Read the model definition and answer for the solid it produces. Units are mm, in the model's axes. Face numbers are marked on the shaded views. A direction names the side the tool comes from. Give positions to 0.01 mm unless a question says otherwise; leave off trailing zeros. Write each loop counter-clockwise with the first axis right and the second up, starting at its lowest first coordinate (ties: lowest second). Pieces come first, ordered by that corner, then holes.
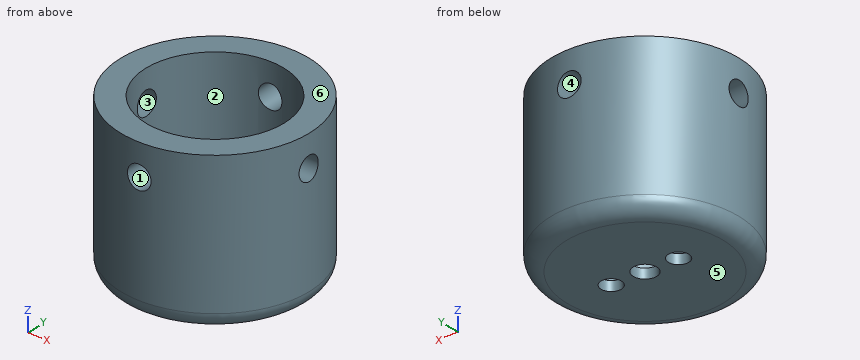
```python
from build123d import *

# Parameters (mm, degrees)
F0_R          = 30.48
F1_DEPTH      = 50.8
F2_R          = 3.81
F3_DEPTH      = 50.801
F4_R          = 3.81
F5_DEPTH      = 30.481
F5_DEPTH_BACK = 30.481
F6_R          = 3.81
F7_DEPTH      = 30.4810001
F7_DEPTH_BACK = 30.4810001
F8_R          = 3.302
F9_DEPTH      = 50.8010001
F10_R         = 22.352
F11_DEPTH     = 47.625
F12_R         = 5.08


with BuildPart() as f1:
    # F0 (on Top) → F1 (new body)
    with BuildSketch(Plane.XY):
        Circle(F0_R)
    extrude(amount=-F1_DEPTH)

    # F2 (on face) → F3 (cut, through all)
    with BuildSketch(Plane(origin=(0, 0, -50.8), x_dir=(1, 0, 0), z_dir=(0, 0, -1))):
        Circle(F2_R)
    extrude(amount=-F3_DEPTH, mode=Mode.SUBTRACT)

    # F4 (on Right) → F5 (cut, two sides)
    with BuildSketch(Plane.YZ) as f5_sk:
        with Locations((0, -10.16)):
            Circle(F4_R)
    extrude(amount=-F5_DEPTH, mode=Mode.SUBTRACT)
    extrude(f5_sk.sketch, amount=F5_DEPTH_BACK, mode=Mode.SUBTRACT)

    # F6 (on Front) → F7 (cut, two sides)
    with BuildSketch(Plane.XZ) as f7_sk:
        with Locations((0, -10.16)):
            Circle(F6_R)
    extrude(amount=-F7_DEPTH, mode=Mode.SUBTRACT)
    extrude(f7_sk.sketch, amount=F7_DEPTH_BACK, mode=Mode.SUBTRACT)

    # F8 (on face) → F9 (cut, through all)
    with BuildSketch(Plane(origin=(0, 0, -50.8), x_dir=(1, 0, 0), z_dir=(0, 0, -1))):
        with Locations((10.922, 0)):
            Circle(F8_R)
        with Locations((-10.8710342307, 0)):
            Circle(F8_R)
    extrude(amount=-F9_DEPTH, mode=Mode.SUBTRACT)

    # F10 (on face) → F11 (cut)
    with BuildSketch(Plane.XY):
        Circle(F10_R)
    extrude(amount=-F11_DEPTH, mode=Mode.SUBTRACT)

    # F12
    f12_edges = [f1.edges().sort_by_distance(p)[0] for p in [
        (-30.48, 0, -50.8),
    ]]
    fillet(f12_edges, radius=F12_R)


solid = f1.part
```
Item 1: Which of the six approach directions +Z, -Z, +X, -X, +Y, -Y give full straight-line access (tool end or side, diameter ignored) to the marked faces 1 and 2?
Result set:
face 1: +Y, -Y
face 2: +Z
Item 2: Section D-D (z = -17.5) is taken. Write down the section's boundary in (x, y).
Result set:
outline: circle Ø60.96 at (0, 0); hole circle Ø44.7 at (0, 0)
Item 3: Each of these flat-tipped pins is pushed along its axis until it touches: pin 1 Ø1.5 at (x, z) = (7, -26.5) entering from -Y; pin 2 Ø9 at (x, z) = (0, -10.16) entering from -Y; pin 3 Ø3 at (x, z) = (-5, -11.5) entering from -Y; pin 4 Ø7.5 at (x, y) = (10.922, 0) entering from +Z (3 decimals). Where does it stop, or does it pass through?
Result set:
pin 1: stops at y = -29.83
pin 2: stops at y = -30.48
pin 3: stops at y = -30.28
pin 4: stops at z = -47.625
Item 4: Section C-C (z = -10.16) is taken. Write down the section's boundary in (x, y), and give its area (3 significant figures).
Result set:
outline: (-30.24, -3.81) arc R30.48 ccw to (-3.81, -30.24) - (-3.81, -22.02) arc R22.35 cw to (-22.02, -3.81) - close; (-30.24, 3.81) - (-22.02, 3.81) arc R22.35 cw to (-3.81, 22.02) - (-3.81, 30.24) arc R30.48 ccw to start; (3.81, -30.24) arc R30.48 ccw to (30.24, -3.81) - (22.02, -3.81) arc R22.35 cw to (3.81, -22.02) - close; (3.81, 22.02) arc R22.35 cw to (22.02, 3.81) - (30.24, 3.81) arc R30.48 ccw to (3.81, 30.24) - close
area: 1,100 mm2
Item 5: Find the intervals of material crossed by line 1 along Y through (x, z) = (-20, -26); line 2 along Y through (x, z) = (5.5, -46.5); line 3 along Z through (x, y) = (-9, -9.5) (3 decimals), in increasing order.
Result set:
line 1: y = -23 to -9.98, 9.98 to 23
line 2: y = -29.92 to -21.66, 21.66 to 29.92
line 3: z = -50.8 to -47.625
Item 6: Determine the mould class of the marked faces 3, 4, 5 and 6 for opening direction Z: pulls with the +Z half, pulls with the -Z half, needs draft (parallel to the pull), parting line crosses it, or undercut.
Result set:
face 3: undercut
face 4: undercut
face 5: pulls with the -Z half
face 6: pulls with the +Z half
Item 7: Section B-B (x = 0) is taken. Write down the section's boundary in (y, z) (3 decimals), and give its area (3 significant figures).
Result set:
outline: (-30.48, -45.72) arc R5.08 ccw to (-25.4, -50.8) - (-3.81, -50.8) - (-3.81, -47.625) - (-22.352, -47.625) - (-22.352, -13.97) - (-30.48, -13.97) - close; (-30.48, -6.35) - (-22.352, -6.35) - (-22.352, 0) - (-30.48, 0) - close; (3.81, -50.8) - (25.4, -50.8) arc R5.08 ccw to (30.48, -45.72) - (30.48, -13.97) - (22.352, -13.97) - (22.352, -47.625) - (3.81, -47.625) - close; (22.352, -6.35) - (30.48, -6.35) - (30.48, 0) - (22.352, 0) - close
area: 809 mm2
Item 8: Section A-A (y = 0) is taken. Give the number of separate pieces and of enclosed holes in the cut face, and give its area (3 significant figures).
Result set:
separate pieces: 6
enclosed holes: 0
area: 767 mm2
